For this review, use the dimensioned drawing (mm, ordinates from the lowest corner) and the shaded views. Coordinates: 2 decimals unless noted, no trailing zeros. Order: outer loops, then holes, each group sorted by start corner. A loop starts at its lowest first (then second) coordinate and runs counter-clockwise, first axis right, second up. Notation, with made-up numbers: (34.5, 17) -> (61.5, 17) arc R19 cw to (61.5, 30) -> close; hole circle Ø11 at (-26, 86.25). An arc over 180 degrees is marked (long way). Use CSV: the item, a comma, the result in double quotes. Start each with the question number.
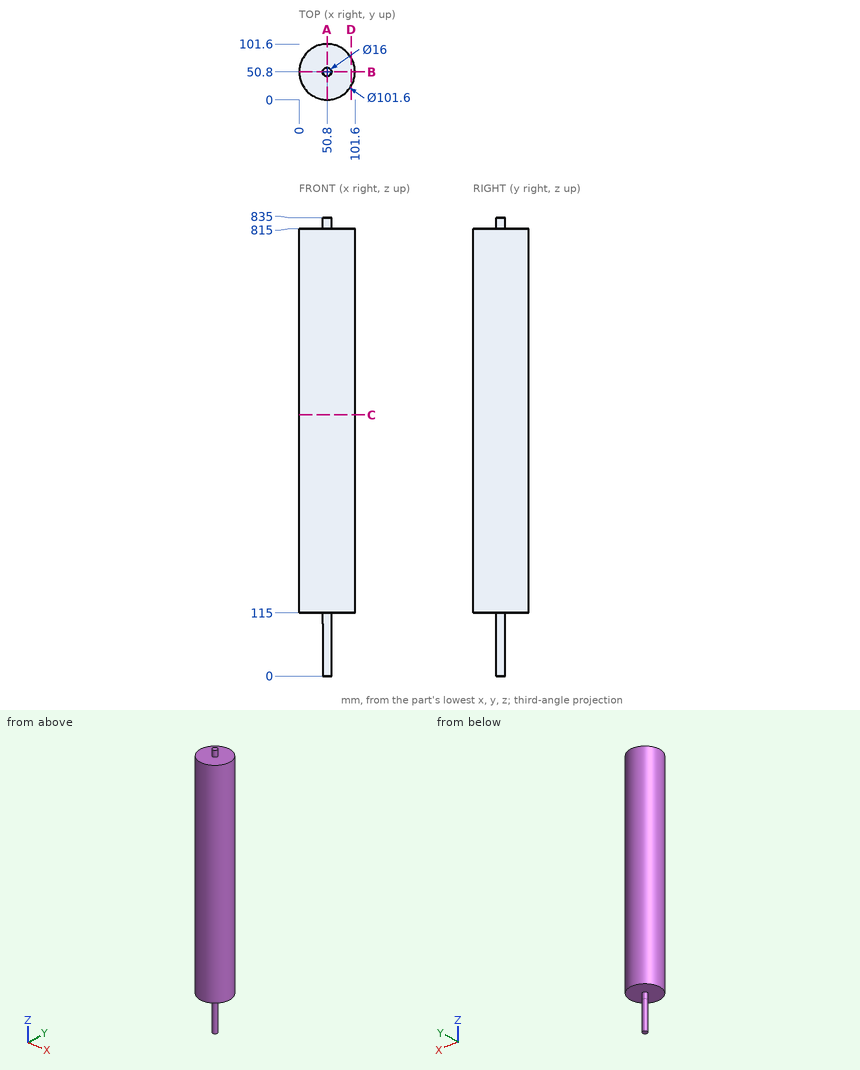
Q1. To check wall thickness, follow probe 1 along Z at (x, y) = (51.5, 9.5); probe 2 along X at (y, z) = (48.5, 720); probe 3 along X at (y, z) = (14, 518). State the ranges of each line that lie inside material, in increasing order.
Q2. Add section C-C, the plane z = 476. State the section outline as (x, y) points.
Q3. Add section A-A, the plane x = 50.8. State the section outline as (y, z) points, then the cut area to 3 significant figures.
Q4. Clearance check with flat-ended pins moving along their axes: pin 1 Ø2 at (x, z) = (80.5, 508.5) entering from +Y; pin 2 Ø8 at (x, z) = (44, 641) entering from -Y; pin 3 Ø6 at (y, z) = (85.5, 220.5) entering from +X. State where each tip first meets the part, or that it passes through.
Q5. Add section D-D, the plane x = 94.5. State the section outline as (y, z) points, then the cut area to 3 significant figures.
Answer block:
1,probe 1,"z = 115 to 815"
1,probe 2,"x = 0.05 to 101.55"
1,probe 3,"x = 15.78 to 85.82"
2,outline,"circle Ø101.6 at (50.8, 50.8)"
3,outline,"(0, 115) -> (42.8, 115) -> (42.8, 0) -> (58.8, 0) -> (58.8, 115) -> (101.6, 115) -> (101.6, 815) -> (58.8, 815) -> (58.8, 835) -> (42.8, 835) -> (42.8, 815) -> (0, 815) -> close"
3,area,"73,300 mm²"
4,pin 1,"stops at y = 92.72"
4,pin 2,"stops at y = 0.08"
4,pin 3,"stops at x = 90.5"
5,outline,"(24.9, 115) -> (76.7, 115) -> (76.7, 815) -> (24.9, 815) -> close"
5,area,"36,300 mm²"
